```python
from build123d import *

# Parameters (mm, degrees)
BOSS_EXTRUDE1_DEPTH = 7.9
SKETCH4_R           = 2.5
CUT_EXTRUDE1_DEPTH  = 8.9
SKETCH_1_R          = 3.5
SKETCH_1_R_2        = 2.5
EXTRUDE_1_DEPTH     = 0.4
SKETCH_2_R          = 3.5
SKETCH_2_R_2        = 2.5
EXTRUDE_2_DEPTH     = 1.7


with BuildPart() as part:
    # Sketch1 → Boss-Extrude1 (new body)
    with BuildSketch(Plane(origin=(0, 0, 0), x_dir=(1, 0, 0), z_dir=(0, 1, 0))):
        Polygon((5.750408681, 0), (2.875204341, 4.98), (-2.875204341, 4.98), (-5.750408681, 0), (-2.875204341, -4.98), (2.875204341, -4.98), align=None)
    extrude(amount=BOSS_EXTRUDE1_DEPTH)

    # Sketch4 → Cut-Extrude1 (cut, through all)
    with BuildSketch(Plane(origin=(0, 7.9, 0), x_dir=(1, 0, 0), z_dir=(0, 1, 0))):
        with Locations((0, -0.79)):
            Circle(SKETCH4_R)
    extrude(amount=-CUT_EXTRUDE1_DEPTH, mode=Mode.SUBTRACT)

    # 草图1 → 凸台-拉伸1 (add)
    with BuildSketch(Plane(origin=(0, 7.9, 0), x_dir=(1, 0, 0), z_dir=(0, 1, 0))):
        with Locations((0, -0.79)):
            Circle(SKETCH_1_R)
        with Locations((0, -0.79)):
            Circle(SKETCH_1_R_2, mode=Mode.SUBTRACT)
    extrude(amount=EXTRUDE_1_DEPTH)

    # 草图2 → 凸台-拉伸2 (add)
    with BuildSketch(Plane.XZ):
        Circle(SKETCH_2_R)
        with Locations((0, 0.79)):
            Circle(SKETCH_2_R_2, mode=Mode.SUBTRACT)
    extrude(amount=EXTRUDE_2_DEPTH)


solid = part.part
```
Part model, mm, in its own coordinate system. A direction names the side the tool comes from. Round coordinates to 2 decimals unless told otherwise and drop trailing zeros. Write each loop counter-clockwise with the first axis right and the second up, starting at its lowest first coordinate (ties: lowest second). Pieces come first, ordered by that corner, then holes. Notation, with made-up numbers: M -7.5,88.25 L 40.5,88.25 A19 ccw 40.5,125.25 Z; hole C -24,49.5 d5. An arc over 180 degrees is marked long. Answer as CSV lines item,"result". Start each with the question number.
1) Band-saw the part on D-D (z = -2). List the corners of the cut face in (x, y), then the cut area to 3 significant figures.
2) Band-saw the part on B-B (x = 0). List the corners of the cut face in (y, z).
3) Mould opens along X. For faces 1 (the face through (-0.54, 3.37, -1.65)), 2 (the face through (-4.293, 3.895, -2.525)), 3 (the face through (-1, 8.3, -2)) say: +X half, -X half, draft (parallel to the pull), parting line (faces both ways), or undercut.
4) Band-saw the part on C-C (z = -1). List the corners of the cut face in (x, y), then the cut area to 3 significant figures.
5) Drill centre lines: L1, parallel to Z at x = 0, y = 0.5; L2, parallel to Y at x = 2.75, z = 2.5; L3, parallel to Z at x = -0.5, y = 1.25. Where is each one in solid material? Low to high.
6) Band-saw the part on A-A (y = 3.25). List the corners of the cut face in (x, z).
7) Which spindle directions (+Z, -Z, +X, -X, +Y, -Y) get a long thin tool onto all of the face, cutting with end or side? Do faces 4 (the face through (0, -1.7, -2)), 5 (the face through (4, 0, 0)), 6 (the face through (3.233, 8.097, 2.131)). Say none if no direction does.
Worked out:
1,outline,"M -4.6,0 L -2.87,0 L -2.87,-1.7 L 2.87,-1.7 L 2.87,0 L 4.6,0 L 4.6,7.9 L 2.11,7.9 L 2.11,8.3 L -2.11,8.3 L -2.11,7.9 L -4.6,7.9 Z"
1,area,"84.1 mm²"
2,outline,"M -1.7,-3.5 L 0,-3.5 L 0,-4.98 L 7.9,-4.98 L 7.9,-2.71 L 8.3,-2.71 L 8.3,-1.71 L -1.7,-1.71 Z; M -1.7,3.29 L 8.3,3.29 L 8.3,4.29 L 7.9,4.29 L 7.9,4.98 L 0,4.98 L 0,3.5 L -1.7,3.5 Z"
3,face 1,"undercut"
3,face 2,"-X half"
3,face 3,"draft"
4,outline,"M -5.17,0 L -3.35,0 L -3.35,-1.7 L -1.75,-1.7 L -1.75,8.3 L -3.01,8.3 L -3.01,7.9 L -5.17,7.9 Z; M 1.75,-1.7 L 3.35,-1.7 L 3.35,0 L 5.17,0 L 5.17,7.9 L 3.01,7.9 L 3.01,8.3 L 1.75,8.3 Z"
4,area,"60.6 mm²"
5,L1,"-4.98 to -1.71, 3.29 to 4.98"
5,L2,"0 to 8.3"
5,L3,"-4.98 to -1.66, 3.24 to 4.98"
6,outline,"M -5.75,0 L -2.88,-4.98 L 2.88,-4.98 L 5.75,0 L 2.88,4.98 L -2.88,4.98 Z; hole C 0,0.79 d5"
7,face 4,"+Z, -Z, +X, -X, -Y"
7,face 5,"-Y"
7,face 6,"+Y"
